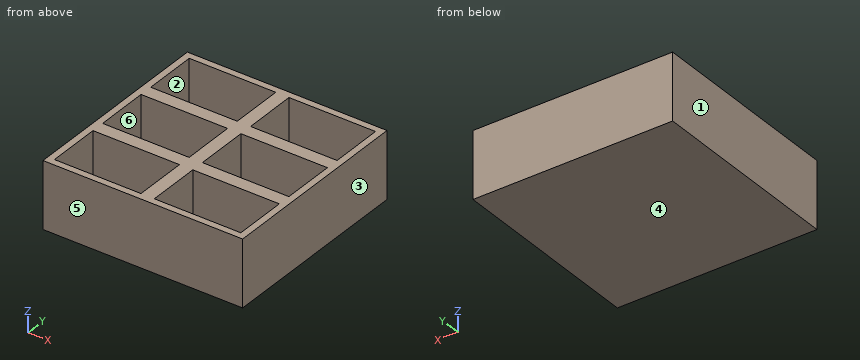
```python
from build123d import *

# Parameters (mm, degrees)
SKETCH_1_W          = 60
SKETCH_1_H          = 60
EXTRUDE_1_DEPTH     = 20
SKETCH_2_W          = 26
SKETCH_2_H          = 16
CUT_EXTRUDE_1_DEPTH = 18


with BuildPart() as part:
    # 草图1 → 凸台-拉伸1 (new body)
    with BuildSketch(Plane.XY):
        with Locations((30, 30)):
            Rectangle(SKETCH_1_W, SKETCH_1_H)
    extrude(amount=-EXTRUDE_1_DEPTH)

    # 草图2 → 切除-拉伸1 (cut)
    with BuildSketch(Plane.XY):
        with Locations((15, 50)):
            Rectangle(SKETCH_2_W, SKETCH_2_H)
        with Locations((45, 50)):
            Rectangle(SKETCH_2_W, SKETCH_2_H)
        with Locations((15, 30)):
            Rectangle(SKETCH_2_W, SKETCH_2_H)
        with Locations((45, 30)):
            Rectangle(SKETCH_2_W, SKETCH_2_H)
        with Locations((15, 10)):
            Rectangle(SKETCH_2_W, SKETCH_2_H)
        with Locations((45, 10)):
            Rectangle(SKETCH_2_W, SKETCH_2_H)
    extrude(amount=-CUT_EXTRUDE_1_DEPTH, mode=Mode.SUBTRACT)


solid = part.part
```
CAD build for the part. Positions are in the model's coordinates, mm. Face numbers are marked on the shaded views. A direction names the side the tool comes from. Round coordinates to 2 decimals unless told otherwise and drop trailing zeros. Order: outer loops, then holes, each group sorted by start corner. A loop starts at its lowest first (then second) coordinate and runs counter-clockwise, first axis right, second up. Notation, with made-up numbers: (87.5, 67.25) -> (116.5, 67.25) arc R32 cw to (116.5, 102.25) -> close; hole circle Ø5 at (56, 53.5). An arc over 180 degrees is marked (long way). Write item = value, one per line.
(1) Cut at A-A (z = -15). Write the cut outline in (x, y), plus the area to 3 significant figures.
Answers follow:
outline = (0, 0) -> (60, 0) -> (60, 60) -> (0, 60) -> close; hole (2, 2) -> (28, 2) -> (28, 18) -> (2, 18) -> close; hole (2, 22) -> (28, 22) -> (28, 38) -> (2, 38) -> close; hole (2, 42) -> (28, 42) -> (28, 58) -> (2, 58) -> close; hole (32, 2) -> (58, 2) -> (58, 18) -> (32, 18) -> close; hole (32, 22) -> (58, 22) -> (58, 38) -> (32, 38) -> close; hole (32, 42) -> (58, 42) -> (58, 58) -> (32, 58) -> close
area = 1,100 mm²
(2) Flat gauge pin, fed straight in: P1, Ø5, axis at x = 14, y = 53, coming from the +Z side. Where does the tip first touch, or does it go through?
Answers follow:
P1 = -18
(3) Drill centre lines: L1, parallel to X at y = 9.5, z = -1.5; L2, parallel to Y at x = 26, z = -16; L3, parallel to Z at x = 11, y = 22.5. Where is each one in solid material? Low to high.
Answers follow:
L1 = 0 to 2, 28 to 32, 58 to 60
L2 = 0 to 2, 18 to 22, 38 to 42, 58 to 60
L3 = -20 to -18
(4) 3-axis set-ups, long thin cutter, end or side, ignore diameter. For the marked faces 5 and 6: which of +Z, -Z, +X, -X, +Y, -Y reach the whole face in a straight line?
Answers follow:
face_5 = +Z, -Z, +X, -X, -Y
face_6 = +Z
(5) Pull direction X, two halves, no side cores. Call the marked faces 1, 2, 3 and 4: +X half, -X half, draft (parallel to the pull), parting line (faces both ways), or undercut.
Answers follow:
face_1 = -X half
face_2 = undercut
face_3 = +X half
face_4 = draft
(6) Cut at B-B (y = 5.5). Write the cut outline in (x, z).
Answers follow:
outline = (0, -20) -> (60, -20) -> (60, 0) -> (58, 0) -> (58, -18) -> (32, -18) -> (32, 0) -> (28, 0) -> (28, -18) -> (2, -18) -> (2, 0) -> (0, 0) -> close
(7) Cut at C-C (x = 25). Write the cut outline in (y, z), plus the area to 3 significant figures.
Answers follow:
outline = (0, -20) -> (60, -20) -> (60, 0) -> (58, 0) -> (58, -18) -> (42, -18) -> (42, 0) -> (38, 0) -> (38, -18) -> (22, -18) -> (22, 0) -> (18, 0) -> (18, -18) -> (2, -18) -> (2, 0) -> (0, 0) -> close
area = 336 mm²
